Source: three-view drawing plus pictorial views. Frame: mm from the lowest corner of the part. Give positions to 0.01 mm unless a question says otherwise; leave off trailing zeros. Loops run counter-clockwise (first coordinate to the right, second up) from the corner with the lowest first, then second, coordinate; pieces in that order, holes last. Notation, with made-up numbers: M 79,33.25 L 136,33.25 A25 ccw 136,52.25 Z; hole C 25,50 d8. An arc over 180 degrees is marked long. Answer as a JSON object with one key per item and string values. Group by question number.
1) Section query C-C on y = 49. Return loops of the section in (x, z).
2) Section query B-B on z = 25. Return loops of the section in (x, y).
3) Draft query along X for the marked faces 1, 2 and 3. Return one class per face: +X half, -X half, draft (parallel to the pull), parting line (faces both ways), or undercut.
4) Ray query, L1, parallel to X at y = 36.5, z = 23; L2, parallel to Z at x = 28.5, y = 63; L3, parallel to Z at x = 19, y = 5. Return the intervals inside material, ascending.
5) Section query A-A on x = 25. Return loops of the section in (y, z), plus the area to 3 significant figures.
6) First-contact query: P1, Ø1.5, axis at y = 54, z = 12.5, coming from the -X side; P2, Ø4, axis at y = 81.5, z = 7, coming from the -X side; P3, Ø1, axis at y = 46, z = 6, coming from the +X side (1 decimal). Flat tips, straight axial feed; report the tip coordinate or a pass-through.
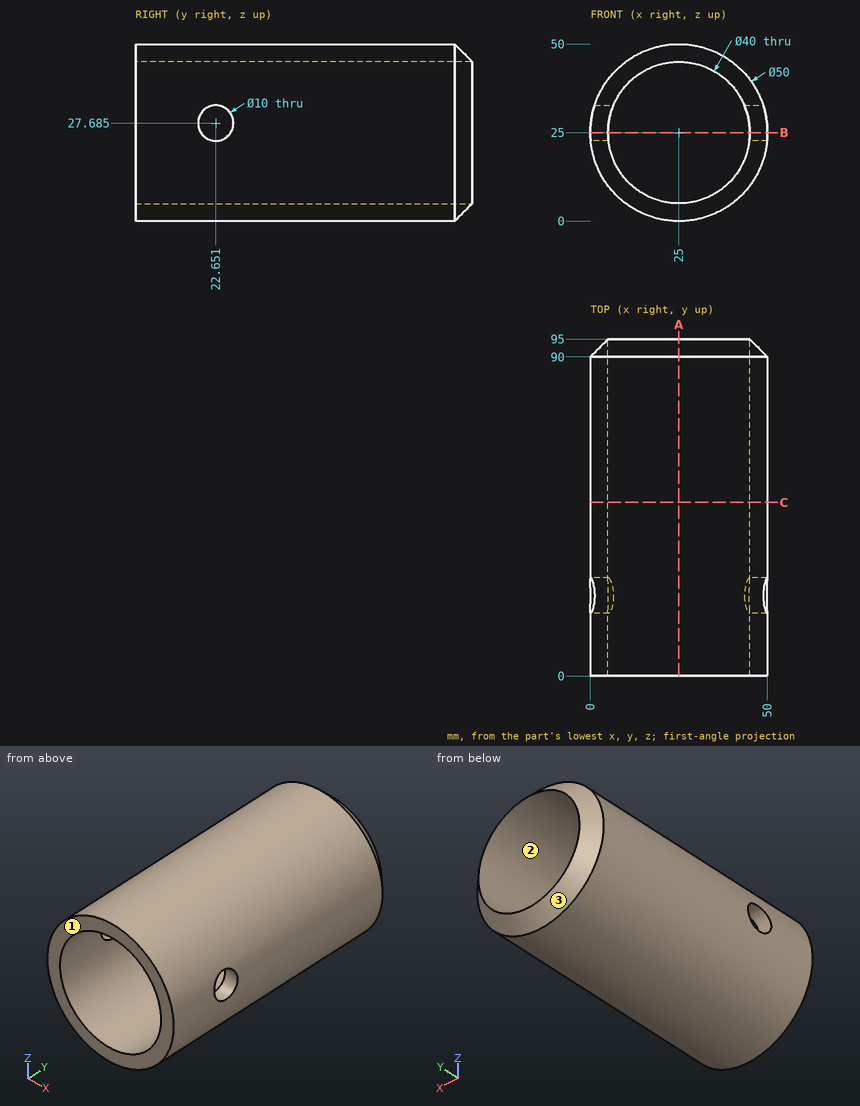
Output:
{
 "1": {"outline": "C 25,25 d50; hole C 25,25 d40"},
 "2": {"outline": "M 0,0 L 5,0 L 5,18.43 L 0,18.43 Z; M 0,26.87 L 5,26.87 L 5,95 L 0,90 Z; M 45,0 L 50,0 L 50,18.43 L 45,18.43 Z; M 45,26.87 L 50,26.87 L 50,90 L 45,95 Z"},
 "3": {"face 1": "draft", "face 2": "undercut", "face 3": "parting line"},
 "4": {"L1": "x = 0.08 to 5.1, 44.9 to 49.92", "L2": "z = 0.25 to 5.31, 44.69 to 49.75", "L3": "z = 0.73 to 5.92, 44.08 to 49.27"},
 "5": {"outline": "M 0,0 L 90,0 L 95,5 L 0,5 Z; M 0,45 L 95,45 L 90,50 L 0,50 Z", "area": "925 mm^2"},
 "6": {"P1": "stops at x = 2.93", "P2": "stops at x = 5.79", "P3": "stops at x = 41.8"}
}
